from build123d import *
from OCP.BRepFilletAPI import BRepFilletAPI_MakeFillet

# Parameters (mm, degrees)
SKETCH1_W               = 6
SKETCH1_H               = 8
BOSS_EXTRUDE1_DEPTH     = 1.5
SKETCH2_W               = 3.4
SKETCH2_H               = 3.6
BOSS_EXTRUDE2_DEPTH     = 1.5
SKETCH3_W               = 10
SKETCH3_H               = 12
BOSS_EXTRUDE3_DEPTH     = 1.5
FILLET1_R1              = 2
FILLET1_R2              = 2.5
CUT_EXTRUDE2_DEPTH      = 21.283244316
CUT_EXTRUDE2_DEPTH_BACK = 21.283244316
SKETCH5_R               = 1.8
CHAMFER3_SIZE           = 1.2


with BuildPart() as part:
    # Sketch1 → Boss-Extrude1 (new, symmetric)
    with BuildSketch(Plane(origin=(0, 0, 0), x_dir=(1, 0, 0), z_dir=(0, 1, 0))):
        Rectangle(SKETCH1_W, SKETCH1_H)
    extrude(amount=BOSS_EXTRUDE1_DEPTH, both=True)

    # Sketch2 → Boss-Extrude2 (add, symmetric)
    with BuildSketch(Plane(origin=(0, 0, 0), x_dir=(1, 0, 0), z_dir=(0, 1, 0))):
        with Locations((0, 5.8)):
            Rectangle(SKETCH2_W, SKETCH2_H)
    extrude(amount=BOSS_EXTRUDE2_DEPTH, both=True)

    # Sketch3 → Boss-Extrude3 (add, symmetric)
    with BuildSketch(Plane(origin=(0, 0, 0), x_dir=(1, 0, 0), z_dir=(0, 1, 0))):
        with Locations((0, 13.6)):
            Rectangle(SKETCH3_W, SKETCH3_H)
    extrude(amount=BOSS_EXTRUDE3_DEPTH, both=True)

    # Fillet1: one fillet with a radius per group of edges: ONE call of the kernel's fillet builder (fillet() takes one radius for all edges)
    fillet1_edges_1 = [part.edges().sort_by_distance(p)[0] for p in [
        (-5, 0, -19.6),
        (5, 0, -19.6),
    ]]
    fillet1_edges_2 = [part.edges().sort_by_distance(p)[0] for p in [
        (-3, 0, 4),
        (3, 0, 4),
    ]]
    fillet1 = BRepFilletAPI_MakeFillet(part.part.solid().wrapped)
    for e in fillet1_edges_1:
        fillet1.Add(FILLET1_R1, e.wrapped)
    for e in fillet1_edges_2:
        fillet1.Add(FILLET1_R2, e.wrapped)
    add(Compound.cast(fillet1.Shape()), mode=Mode.REPLACE)

    # Sketch5 → Cut-Extrude2 (cut, two sides: drawn at the far end of the back side and taken through both)
    with BuildSketch(Plane(origin=(0, 0, 0), x_dir=(1, 0, 0), z_dir=(0, 1, 0)).offset(-CUT_EXTRUDE2_DEPTH_BACK)):
        with Locations(Location((0, 16.3, 0), (0, 0, 270))):
            Circle(SKETCH5_R)
        with BuildLine():
            Line((-1.65, -1.1), (-1.65, 1.1))
            ThreePointArc((-1.65, 1.1), (0, 2.75), (1.65, 1.1))
            Line((1.65, 1.1), (1.65, -1.1))
            ThreePointArc((1.65, -1.1), (0, -2.75), (-1.65, -1.1))
        make_face()
    extrude(amount=CUT_EXTRUDE2_DEPTH + CUT_EXTRUDE2_DEPTH_BACK, mode=Mode.SUBTRACT)

    # Chamfer3
    # the kernel refuses this chamfer: 1.2 mm, written as the material it takes off along each edge
    with BuildSketch(Plane(origin=(8.086019586, -1.5, -7.6), x_dir=(0, 0.9996219169112968, 0.027495876610586632), z_dir=(-1, 0, 0)), Plane(origin=(-1.7, -1.5, -7.6), x_dir=(0, 0.9996219169112968, 0.027495876610586632), z_dir=(-1, 0, 0)), Plane(origin=(-1.7, 1.5, -7.6), x_dir=(0, 0.027495876610586483, -0.9996219169112968), z_dir=(-1, 0, 0)), Plane(origin=(8.086019586, 1.5, -7.6), x_dir=(0, 0.027495876610586483, -0.9996219169112968), z_dir=(-1, 0, 0))) as chamfer3_piece_1:
        Polygon((CHAMFER3_SIZE * 0.999621916911, CHAMFER3_SIZE * 0.0274958766106), (-CHAMFER3_SIZE * 0.0274958766106, CHAMFER3_SIZE * 0.999621916911), (0, 0), align=None)
    extrude(amount=6.386019586, mode=Mode.SUBTRACT)
    with BuildSketch(Plane(origin=(5, -1.5, -20.686019586), x_dir=(0.027495876610586632, 0.9996219169112968, 0), z_dir=(0, 0, 1)), Plane(origin=(5, 1.5, -20.686019586), x_dir=(-0.9996219169112968, 0.027495876610586452, 0), z_dir=(0, 0, 1)), Plane(origin=(-5, -1.5, -4.513980414), x_dir=(-0.027495876610586632, 0.9996219169112968, 0), z_dir=(0, 0, -1)), Plane(origin=(-5, 1.5, -4.513980414), x_dir=(0.9996219169112968, 0.027495876610586452, 0), z_dir=(0, 0, -1))) as chamfer3_piece_2:
        Polygon((CHAMFER3_SIZE * 0.999621916911, CHAMFER3_SIZE * 0.0274958766106), (-CHAMFER3_SIZE * 0.0274958766106, CHAMFER3_SIZE * 0.999621916911), (0, 0), align=None)
    extrude(amount=16.172039171, mode=Mode.SUBTRACT)


solid = part.part
Model file for the job. Use its own axes, mm. A direction names the side the tool comes from. Give positions to 0.01 mm unless a question says otherwise; leave off trailing zeros. Write each loop counter-clockwise with the first axis right and the second up, starting at its lowest first coordinate (ties: lowest second). Pieces come first, ordered by that corner, then holes. Notation, with made-up numbers: (25, -22.5) -> (35, -22.5) arc R26 cw to (35, 14.5) -> close; hole circle Ø11 at (48, -40). An arc over 180 degrees is marked (long way). Write item = value, one per line.
(1) Slice it at A-A, the plane x = 0. Give the cut face in (y, z), then the cut area to 3 significant figures.
Determined:
outline = (-1.5, -19.6) -> (1.5, -19.6) -> (1.5, -18.1) -> (-1.5, -18.1) -> close; (-1.5, -14.5) -> (1.5, -14.5) -> (1.5, -2.75) -> (-1.5, -2.75) -> close; (-1.5, 2.75) -> (1.5, 2.75) -> (1.5, 4) -> (-1.5, 4) -> close
area = 43.5 mm2
(2) Slice it at C-C, the plane z = -15.25. Give the cut face in (x, y), then the cut area to 3 significant figures.
Determined:
outline = (-5, -0.3) -> (-3.8, -1.5) -> (-1.46, -1.5) -> (-1.46, 1.5) -> (-3.8, 1.5) -> (-5, 0.3) -> close; (1.46, -1.5) -> (3.8, -1.5) -> (5, -0.3) -> (5, 0.3) -> (3.8, 1.5) -> (1.46, 1.5) -> close
area = 18.3 mm2
(3) Flat gauge pins, fed straight in: P1, Ø3, axis at x = 0, z = -16.3, coming from the -Y side; P2, Ø1.5, axis at x = 2.5, z = -8.5, coming from the -Y side; P3, Ø1.1, axis at y = 0.5, z = 0, coming from the +X side; P4, Ø1.8, axis at y = -0.5, z = 0.5, coming from the -X side. Where does each tip first touch, or does it go through?
Determined:
P1 = through
P2 = -1.5
P3 = 3
P4 = -3
(4) Mould opens along Z. For faces 1 (the face through (3, 0, -1)), 2 (the face through (-2.287, 0.021, 3.248)), 3 (the face through (-2, 0, -4)) say: released by +Z, released by -Z, zero draft, split by the parting line, or undercut.
Determined:
face_1 = zero draft
face_2 = released by +Z
face_3 = undercut
(5) Slice it at B-B, the plane y = -1.2. Give the cut face in (x, z), then the cut area to 3 significant figures.
Determined:
outline = (-4.1, -19.27) arc R2 ccw to (-3, -19.6) -> (3, -19.6) arc R2 ccw to (4.1, -19.27) -> (4.1, -8.5) -> (1.7, -8.5) -> (1.7, -4) -> (3, -4) -> (3, 1.5) arc R2.5 ccw to (0.5, 4) -> (-0.5, 4) arc R2.5 ccw to (-3, 1.5) -> (-3, -4) -> (-1.7, -4) -> (-1.7, -8.5) -> (-4.1, -8.5) -> close; hole circle Ø3.6 at (0, -16.3); hole (-1.65, -1.1) arc R1.65 ccw to (1.65, -1.1) -> (1.65, 1.1) arc R1.65 ccw to (-1.65, 1.1) -> close
area = 125 mm2
(6) Slice it at D-D, the plane x = -2.75. Give the cut face in (y, z), then the cut area to 3 significant figures.
Determined:
outline = (-1.5, -19.6) -> (1.5, -19.6) -> (1.5, -8.8) -> (0.3, -7.6) -> (-0.3, -7.6) -> (-1.5, -8.8) -> close; (-1.5, -4) -> (1.5, -4) -> (1.5, 2.59) -> (-1.5, 2.59) -> close
area = 54.3 mm2
(7) Probe line 1 along Z through (x, y) = (0, 0.2); line 2 along X through (y, z) = (0, -16.3); line 3 along X through (y, z) = (0.45, -1). List the from-to ranges inside material, lowest first.
Determined:
line_1 = -19.6 to -18.1, -14.5 to -2.75, 2.75 to 4
line_2 = -5 to -1.8, 1.8 to 5
line_3 = -3 to -1.65, 1.65 to 3
(8) Tool access for faces 4 (the face through (0.04, -0.02, 2.75)), 5 (the face through (-3, 0.9, -8.2)), 6 (the face through (2, 0, -4)), 7 (the face through (3, 0.9, -8.2)): list every direction of +Z, -Z, +X, -X, +Y, -Y with a clear straight run to the whole face (end or side of a thin tool).
Determined:
face_4 = +Y, -Y
face_5 = -X, +Y
face_6 = +X, +Y, -Y
face_7 = +X, +Y
